Work out the finished part from the listing and answer in its coordinate system (mm). Face numbers are marked on the shaded views. A direction names the side the tool comes from. Coordinates: 2 decimals unless noted, no trailing zeros. Order: outer loops, then holes, each group sorted by start corner. A loop starts at its lowest first (then second) coordinate and runs counter-clockwise, first axis right, second up.
1. The part is cut by section D-D, the plane y = -0.75. Give the vertices of the cut face in (x, z), then the cut area to 3 significant figures.
2. The part is cut by section C-C, the plane x = 23.55. Give the vertices of the cut face in (y, z), then the cut area to 3 significant figures.
3. Flat-ended cylindrical pins translate along their axes: pin 1 Ø14.5 at (x, z) = (0, 0) entering from +Y; pin 2 Ø1 at (x, y) = (22.5, 0) entering from +Z. Find the tip coordinate at first contact, or state that the pin passes through.
4. The part is cut by section B-B, the plane x = 0. Give the vertices of the cut face in (y, z).
5. The part is cut by section A-A, the plane z = 0. Give the vertices of the cut face in (x, y).
6. A tool of negligible diameter and unlimited length cuts with its end or side. For the marked faces 1 and 2, from which of +Z, -Z, +X, -X, +Y, -Y can it reach the whole face along a straight path? Write none if from no direction.
7. Find the intervals of material crossed by probe 1 along Z at (x, y) = (-25.5, 0.1); probe 2 along Z at (x, y) = (0, -1.3); probe 3 along Y at (x, z) = (25, -2), in increasing order.
8. Determine the mould class of the marked faces 3 and 4 for opening direction Z: +Z half, -Z half, draft (parallel to the pull), parting line (faces both ways), or undercut.
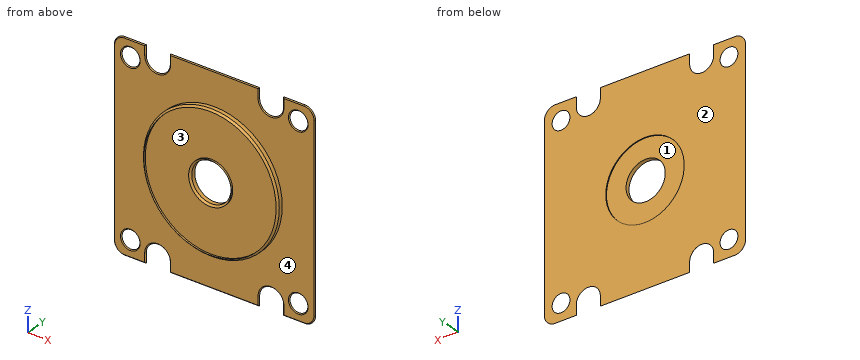
```python
from build123d import *

# Parameters (mm, degrees)
SKETCH036_R     = 5.5
PAD020_DEPTH    = 6
SKETCH035_R     = 5.5
PAD019_DEPTH    = 5
SKETCH037_R     = 19.05
SKETCH037_R_2   = 5.5
PAD021_DEPTH    = 1.6
SKETCH038_R     = 2.5
POCKET015_DEPTH = 11.001
SKETCH039_R     = 1.5
POCKET016_DEPTH = 12.601
POCKET017_DEPTH = 3
SKETCH041_R     = 11
POCKET018_DEPTH = 11
CHAMFER004_SIZE = 0.25
CHAMFER005_SIZE = 0.5
SKETCH042_R     = 40.822693
POCKET022_DEPTH = 10.75
SKETCH043_R     = 18.55
SKETCH043_R_2   = 6
POCKET023_DEPTH = 0.5


with BuildPart() as part:
    # Sketch036 → Pad020 (new body)
    with BuildSketch(Plane(origin=(0, 5, 0), x_dir=(1, 0, 0), z_dir=(0, 1, 0))):
        with BuildLine():
            Line((-26.2, 19.45), (-23.7, 19.45))
            ThreePointArc((-23.7, 19.45), (-20.694796, 20.694796), (-19.45, 23.7))
            Line((-19.45, 23.7), (-19.45, 26.2))
            ThreePointArc((-17.45, 28.2), (-18.864214, 27.614214), (-19.45, 26.2))
            Line((-17.45, 28.2), (17.45, 28.2))
            ThreePointArc((19.45, 26.2), (18.864214, 27.614214), (17.45, 28.2))
            Line((19.45, 26.2), (19.45, 23.7))
            ThreePointArc((19.45, 23.7), (20.694796, 20.694796), (23.7, 19.45))
            Line((23.7, 19.45), (26.2, 19.45))
            ThreePointArc((28.2, 17.45), (27.614214, 18.864214), (26.2, 19.45))
            Line((28.2, 17.45), (28.2, -17.45))
            ThreePointArc((26.2, -19.45), (27.614214, -18.864214), (28.2, -17.45))
            Line((23.7, -19.45), (26.2, -19.45))
            ThreePointArc((23.7, -19.45), (20.694796, -20.694796), (19.45, -23.7))
            Line((19.45, -26.2), (19.45, -23.7))
            ThreePointArc((17.45, -28.2), (18.864214, -27.614214), (19.45, -26.2))
            Line((-17.45, -28.2), (17.45, -28.2))
            ThreePointArc((-19.45, -26.2), (-18.864214, -27.614214), (-17.45, -28.2))
            Line((-19.45, -26.2), (-19.45, -23.7))
            ThreePointArc((-19.45, -23.7), (-20.694796, -20.694796), (-23.7, -19.45))
            Line((-26.2, -19.45), (-23.7, -19.45))
            ThreePointArc((-28.2, -17.45), (-27.614214, -18.864214), (-26.2, -19.45))
            Line((-28.2, 17.45), (-28.2, -17.45))
            ThreePointArc((-26.2, 19.45), (-27.614214, 18.864214), (-28.2, 17.45))
        make_face()
        Circle(SKETCH036_R, mode=Mode.SUBTRACT)
    extrude(amount=PAD020_DEPTH)

    # Sketch035 (on Face26 of Pad020) → Pad019 (join)
    with BuildSketch(Plane.XZ.offset(-5)):
        with BuildLine():
            Line((-28.2, 25.2), (-28.2, -25.2))
            ThreePointArc((-28.2, -25.2), (-27.32132, -27.32132), (-25.2, -28.2))
            Line((-25.2, -28.2), (25.2, -28.2))
            ThreePointArc((25.2, -28.2), (27.32132, -27.32132), (28.2, -25.2))
            Line((28.2, 25.2), (28.2, -25.2))
            ThreePointArc((28.2, 25.2), (27.32132, 27.32132), (25.2, 28.2))
            Line((-25.2, 28.2), (25.2, 28.2))
            ThreePointArc((-25.2, 28.2), (-27.32132, 27.32132), (-28.2, 25.2))
        make_face()
        Circle(SKETCH035_R, mode=Mode.SUBTRACT)
    extrude(amount=PAD019_DEPTH)

    # Sketch037 (on Face33 of Pad019) → Pad021 (join)
    with BuildSketch(Plane.XZ):
        Circle(SKETCH037_R)
        Circle(SKETCH037_R_2, mode=Mode.SUBTRACT)
    extrude(amount=PAD021_DEPTH)

    # Sketch038 (on Face33 of Pad021) → Pocket015 (cut, through all)
    with BuildSketch(Plane.XZ):
        with Locations((-23.55, 23.55)):
            Circle(SKETCH038_R)
        with Locations((23.55, 23.55)):
            Circle(SKETCH038_R)
        with Locations((23.55, -23.55)):
            Circle(SKETCH038_R)
        with Locations((-23.55, -23.55)):
            Circle(SKETCH038_R)
    extrude(amount=-POCKET015_DEPTH, mode=Mode.SUBTRACT)

    # Sketch039 (on Face5 of Pocket015) → Pocket016 (cut, through all)
    with BuildSketch(Plane(origin=(0, 11, 0), x_dir=(1, 0, 0), z_dir=(0, 1, 0))):
        with Locations((-15.9, 25.5)):
            Circle(SKETCH039_R)
        with Locations((15.9, 25.5)):
            Circle(SKETCH039_R)
        with Locations((-15.9, -25.5)):
            Circle(SKETCH039_R)
        with Locations((15.9, -25.5)):
            Circle(SKETCH039_R)
    extrude(amount=-POCKET016_DEPTH, mode=Mode.SUBTRACT)

    # Sketch040 (on Face38 of Pocket016) → Pocket017 (cut)
    with BuildSketch(Plane.XZ):
        with BuildLine():
            Line((-19.275, -25.5), (-19.275, -30.5))
            Line((-19.275, -30.5), (-12.525, -30.5))
            Line((-12.525, -30.5), (-12.525, -25.5))
            ThreePointArc((-12.525, -25.5), (-15.9, -22.125), (-19.275, -25.5))
        make_face()
        with BuildLine():
            Line((12.525, -25.5), (12.525, -30.5))
            Line((12.525, -30.5), (19.275, -30.5))
            Line((19.275, -30.5), (19.275, -25.5))
            ThreePointArc((19.275, -25.5), (15.9, -22.125), (12.525, -25.5))
        make_face()
        with BuildLine():
            Line((-19.275, 25.5), (-19.275, 30.5))
            Line((-19.275, 30.5), (-12.525, 30.5))
            Line((-12.525, 30.5), (-12.525, 25.5))
            ThreePointArc((-19.275, 25.5), (-15.9, 22.125), (-12.525, 25.5))
        make_face()
        with BuildLine():
            Line((12.525, 25.5), (12.525, 30.5))
            Line((12.525, 30.5), (19.275, 30.5))
            Line((19.275, 30.5), (19.275, 25.5))
            ThreePointArc((12.525, 25.5), (15.9, 22.125), (19.275, 25.5))
        make_face()
    extrude(amount=-POCKET017_DEPTH, mode=Mode.SUBTRACT)

    # Sketch041 (on Face5 of Pocket017) → Pocket018 (cut)
    with BuildSketch(Plane(origin=(0, 11, 0), x_dir=(1, 0, 0), z_dir=(0, 1, 0))):
        Circle(SKETCH041_R)
    extrude(amount=-POCKET018_DEPTH, mode=Mode.SUBTRACT)

    # Chamfer004
    chamfer004_edges = [part.edges().sort_by_distance(p)[0] for p in [
        (-28.2, 0, 0),
        (-27.32132, 0, 27.32132),
        (-26.05, 0, 23.55),
        (-22.2375, 0, 28.2),
        (-15.9, 0, 22.125),
        (0, 0, 28.2),
        (15.9, 0, 22.125),
        (21.05, 0, 23.55),
        (28.2, 0, 0),
        (-27.32132, 0, -27.32132),
        (-22.2375, 0, -28.2),
        (-26.05, 0, -23.55),
        (-15.9, 0, -22.125),
        (0, 0, -28.2),
        (27.32132, 0, -27.32132),
        (22.2375, 0, -28.2),
        (21.05, 0, -23.55),
        (15.9, 0, -22.125),
    ]]
    chamfer(chamfer004_edges, length=CHAMFER004_SIZE)

    # Chamfer005
    chamfer005_edges = [part.edges().sort_by_distance(p)[0] for p in [
        (-19.05, -1.6, 0),
        (-5.5, -1.6, 0),
    ]]
    chamfer(chamfer005_edges, length=CHAMFER005_SIZE)

    # Sketch042 (on Face7 of Pocket018) → Pocket022 (cut)
    with BuildSketch(Plane(origin=(0, 11, 0), x_dir=(1, 0, 0), z_dir=(0, 1, 0))):
        Circle(SKETCH042_R)
    extrude(amount=-POCKET022_DEPTH, mode=Mode.SUBTRACT)

    # Sketch043 (on Face4 of Pocket022) → Pocket023 (cut)
    with BuildSketch(Plane.XZ.offset(1.6)):
        Circle(SKETCH043_R)
        Circle(SKETCH043_R_2, mode=Mode.SUBTRACT)
    extrude(amount=-POCKET023_DEPTH, mode=Mode.SUBTRACT)


solid = part.part
```
Geometry says:
1. outline: circle Ø38.1 at (0, 0); hole circle Ø11 at (0, 0)
1. area: 1,050 mm2
2. outline: (0, -27.95) - (0.25, -28.2) - (0.25, -26.05) - (0, -26.3) - close; (0, -20.8) - (0.25, -21.05) - (0.25, 21.05) - (0, 20.8) - close; (0, 26.3) - (0.25, 26.05) - (0.25, 28.2) - (0, 27.95) - close
2. area: 11.4 mm2
3. pin 1: stops at y = 0
3. pin 2: stops at z = 28.2
4. outline: (-1.6, -18.55) - (-1.1, -19.05) - (0, -19.05) - (0, -27.95) - (0.25, -28.2) - (0.25, -11) - (0, -11) - (0, -5.5) - (-1.1, -5.5) - (-1.6, -6) - (-1.1, -6) - (-1.1, -18.55) - close; (-1.6, 6) - (-1.1, 5.5) - (0, 5.5) - (0, 11) - (0.25, 11) - (0.25, 28.2) - (0, 27.95) - (0, 19.05) - (-1.1, 19.05) - (-1.6, 18.55) - (-1.1, 18.55) - (-1.1, 6) - close
5. outline: (-28.2, 0.25) - (-27.95, 0) - (-19.05, 0) - (-19.05, -1.1) - (-18.55, -1.6) - (-18.55, -1.1) - (-6, -1.1) - (-6, -1.6) - (-5.5, -1.1) - (-5.5, 0) - (-11, 0) - (-11, 0.25) - close; (5.5, -1.1) - (6, -1.6) - (6, -1.1) - (18.55, -1.1) - (18.55, -1.6) - (19.05, -1.1) - (19.05, 0) - (27.95, 0) - (28.2, 0.25) - (11, 0.25) - (11, 0) - (5.5, 0) - close
6. face 1: +Y
6. face 2: +Z, -Z, +X, -X, +Y
7. probe 1: z = -28.03 to -25.34, -21.76 to 21.76, 25.34 to 28.03
7. probe 2: z = -18.85 to -18.55, -6 to -5.7, 5.7 to 6, 18.55 to 18.85
7. probe 3: y = 0 to 0.25
8. face 3: undercut
8. face 4: draft
